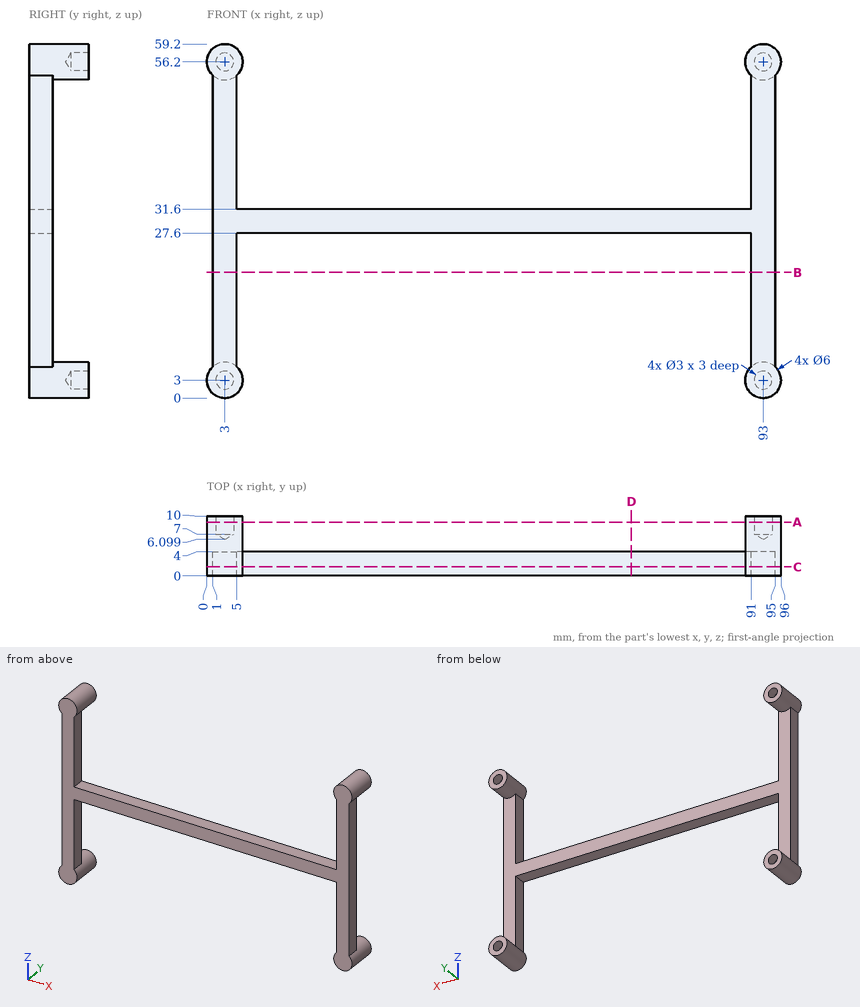
Here's the drawing with two shaded views (mm, measured from the low corner). I have some questions. Coordinates: 2 decimals unless noted, no trailing zeros. Write each loop counter-clockwise with the first axis right and the second up, starting at its lowest first coordinate (ties: lowest second). Pieces come first, ordered by that corner, then holes.
Item 1: I want a section at B-B on z = 21. Write out the boundary of the cut face in (x, y).
Item 2: I want a section at C-C on y = 1.5. Write out the boundary of the cut face in (x, z).
Item 3: I want a section at D-D on x = 71. Write out the boundary of the cut face in (y, z).
Item 4: Will these pins go through, and if not, where does the flat tip stop? pin 1 (4.5 mm diameter, centred on x = 60.5, y = 2, fed in from +Z); pin 2 (1.2 mm diameter, centred on y = 2, z = 48, fed in from -X); pin 3 (3 mm diameter, centred on y = 1.5, z = 15, fed in from +X).
Item 5: I want a section at A-A on y = 9. Write out the boundary of the cut face in (x, z).
Item 6: If I drill on line 1 (Z direction, x = 3, y = 7.9); line 2 (X direction, y = 8.55, z = 56.2); line 3 (X direction, y = 2, z = 35.5), over which ranges is the centre line in solid material (lowest first)?
Findings below:
1. outline: (1, 0) - (5, 0) - (5, 4) - (1, 4) - close; (91, 0) - (95, 0) - (95, 4) - (91, 4) - close
2. outline: (1, 5.24) arc R3 ccw (long way) to (5, 5.24) - (5, 27.6) - (91, 27.6) - (91, 5.24) arc R3 ccw (long way) to (95, 5.24) - (95, 53.96) arc R3 ccw (long way) to (91, 53.96) - (91, 31.6) - (5, 31.6) - (5, 53.96) arc R3 ccw (long way) to (1, 53.96) - close
3. outline: (0, 27.6) - (4, 27.6) - (4, 31.6) - (0, 31.6) - close
4. pin 1: stops at z = 31.6
4. pin 2: stops at x = 1
4. pin 3: stops at x = 95
5. outline: circle Ø6 at (3, 3); circle Ø6 at (3, 56.2); circle Ø6 at (93, 3); circle Ø6 at (93, 56.2); hole circle Ø3 at (3, 3); hole circle Ø3 at (3, 56.2); hole circle Ø3 at (93, 3); hole circle Ø3 at (93, 56.2)
6. line 1: z = 0 to 1.5, 4.5 to 6, 53.2 to 54.7, 57.7 to 59.2
6. line 2: x = 0 to 1.5, 4.5 to 6, 90 to 91.5, 94.5 to 96
6. line 3: x = 1 to 5, 91 to 95
